from build123d import *

# Parameters (mm, degrees)
F1_DEPTH = 19.05
F2_R     = 50.8
F2_W     = 76.2
F2_H     = 76.2
F2_W_2   = 406.4
F2_H_2   = 144.050563
F3_DEPTH = 19.051
F4_W     = 58.42
F4_H     = 58.42
F4_W_2   = 76.2
F4_H_2   = 254
F5_DEPTH = 6.35
F2_W_3   = 127
F2_H_3   = 59.149437
F6_DEPTH = 19.051


with BuildPart() as f1:
    # F0 (on Front) → F1 (new body)
    with BuildSketch(Plane.XZ):
        with BuildLine():
            Line((298.45, 711.2), (-298.45, 711.2))
            ThreePointArc((-298.45, 711.2), (-302.940128, 709.340128), (-304.8, 704.85))
            Line((-304.8, 704.85), (-304.8, 406.4))
            ThreePointArc((-304.8, 406.4), (-177.8, 127), (-304.8, -152.4))
            Line((-304.8, -152.4), (-304.8, -704.85))
            ThreePointArc((-304.8, -704.85), (-302.940128, -709.340128), (-298.45, -711.2))
            Line((-298.45, -711.2), (298.45, -711.2))
            ThreePointArc((298.45, -711.2), (302.940128, -709.340128), (304.8, -704.85))
            Line((304.8, -704.85), (304.8, -152.4))
            ThreePointArc((304.8, -152.4), (177.8, 127), (304.8, 406.4))
            Line((304.8, 406.4), (304.8, 704.85))
            ThreePointArc((304.8, 704.85), (302.940128, 709.340128), (298.45, 711.2))
        make_face()
    extrude(amount=F1_DEPTH)

    # F2 (on face) → F3 (cut, through all)
    with BuildSketch(Plane.XZ.offset(19.05)):
        with Locations((0, 355.6)):
            Circle(F2_R)
        with Locations((228.878711, -255.543973)):
            Rectangle(F2_W, F2_H)
        with Locations((0, -541.925281)):
            Rectangle(F2_W_2, F2_H_2)
    extrude(amount=-F3_DEPTH, mode=Mode.SUBTRACT)

    # F4 (on face) → F5 (cut)
    with BuildSketch(Plane.XZ):
        with Locations((123.19, -662.210563)):
            Rectangle(F4_W, F4_H)
        with Locations((-123.19, -662.210563)):
            Rectangle(F4_W, F4_H)
        with Locations((133.35, 355.6)):
            Rectangle(F4_W_2, F4_H_2)
        with Locations((-133.35, 355.6)):
            Rectangle(F4_W_2, F4_H_2)
    extrude(amount=F5_DEPTH, mode=Mode.SUBTRACT)

    # F2 (on face) → F6 (cut, through all)
    with BuildSketch(Plane.XZ.offset(19.05)):
        with Locations((0, -662.575281)):
            Rectangle(F2_W_3, F2_H_3)
    extrude(amount=-F6_DEPTH, mode=Mode.SUBTRACT)


solid = f1.part
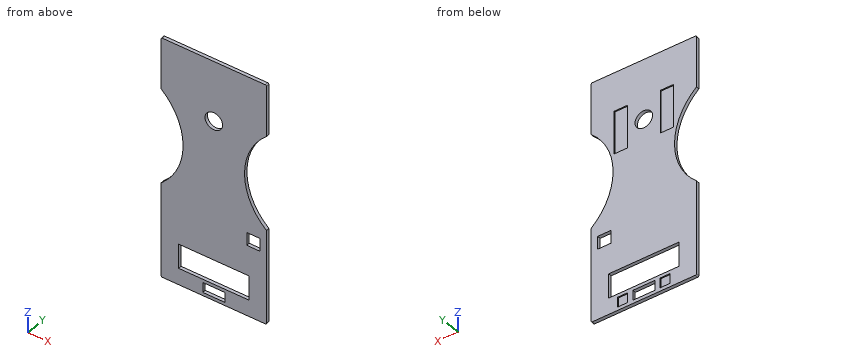
Here's how the part is built. I have some questions about the finished solid (model axes, mm). Coordinates: 2 decimals unless noted, no trailing zeros. Order: outer loops, then holes, each group sorted by start corner. A loop starts at its lowest first (then second) coordinate and runs counter-clockwise, first axis right, second up.
Item 1: For P1, Ø1.9, axis at y = -2.5, z = 382.5, coming from the +X side; P2, Ø5, axis at y = -14.5, z = 379.5, coming from the +X side; P3, Ø1.9, axis at y = -2.5, z = 383, coming from the +X side, each with a flat end and sliding along its axis, tell me the tip position at first contact or that it passes through.
Result sheet:
P1: stops at x = 280.77
P2: stops at x = 279.39
P3: stops at x = 281.25
Item 2: If we section it at D-D on x = -127.5: List the corners of the cut face in (y, z) for me, plus the area to 3 significant figures.
Result sheet:
outline: (-19.05, -711.2) - (0, -711.2) - (0, -691.42) - (-6.35, -691.42) - (-6.35, -633) - (0, -633) - (0, -613.95) - (-19.05, -613.95) - close; (-19.05, -469.9) - (0, -469.9) - (0, 228.6) - (-6.35, 228.6) - (-6.35, 482.6) - (0, 482.6) - (0, 711.2) - (-19.05, 711.2) - close
area: 22,400 mm2
Item 3: I need wall thicknesses on line 1 (Z direction, x = 0, y = -13.5); line 2 (Z direction, x = -164, y = -3.75); line 3 (X direction, y = -5.75, z = 425.5). Which ranges of each line are inside material? Lowest first, please.
Result sheet:
line 1: z = -711.2 to -692.15, -633 to -613.95, -469.9 to 304.8, 406.4 to 711.2
line 2: z = -711.2 to -613.95, -469.9 to 228.6, 482.6 to 711.2
line 3: x = -304.8 to -171.45, -95.25 to 95.25, 171.45 to 304.8
Item 4: If we section it at B-B on x = 0: List the corners of the cut face in (y, z) for me.
Result sheet:
outline: (-19.05, -711.2) - (0, -711.2) - (0, -692.15) - (-19.05, -692.15) - close; (-19.05, -633) - (0, -633) - (0, -613.95) - (-19.05, -613.95) - close; (-19.05, -469.9) - (0, -469.9) - (0, 304.8) - (-19.05, 304.8) - close; (-19.05, 406.4) - (0, 406.4) - (0, 711.2) - (-19.05, 711.2) - close
Item 5: If we section it at C-C on y = -12: List the corners of the cut face in (x, z) for me.
Result sheet:
outline: (-304.8, -704.85) arc R6.35 ccw to (-298.45, -711.2) - (298.45, -711.2) arc R6.35 ccw to (304.8, -704.85) - (304.8, -152.4) arc R370.84 cw to (304.8, 406.4) - (304.8, 704.85) arc R6.35 ccw to (298.45, 711.2) - (-298.45, 711.2) arc R6.35 ccw to (-304.8, 704.85) - (-304.8, 406.4) arc R370.84 cw to (-304.8, -152.4) - close; hole (-203.2, -613.95) - (203.2, -613.95) - (203.2, -469.9) - (-203.2, -469.9) - close; hole (-63.5, -692.15) - (63.5, -692.15) - (63.5, -633) - (-63.5, -633) - close; hole circle Ø101.6 at (0, 355.6); hole (190.78, -293.64) - (266.98, -293.64) - (266.98, -217.44) - (190.78, -217.44) - close
Item 6: If we section it at A-A on z = -582: List the corners of the cut face in (x, y) for me, plus the area to 3 significant figures.
Result sheet:
outline: (-304.8, -19.05) - (-203.2, -19.05) - (-203.2, 0) - (-304.8, 0) - close; (203.2, -19.05) - (304.8, -19.05) - (304.8, 0) - (203.2, 0) - close
area: 3,870 mm2
